Verification items for the finished model (mm, model axes). Round coordinates to 2 decimals unless told otherwise and drop trailing zeros. Order: outer loops, then holes, each group sorted by start corner. A loop starts at its lowest first (then second) coordinate and runs counter-clockwise, first axis right, second up. Notation, with made-up numbers: M 62.5,80 L 70.5,80 A27 ccw 70.5,116 Z; hole C 29.25,20 d6. An arc over 180 degrees is marked long. Write item = value, one per line. Start each with the question number.
from build123d import *


with BuildPart() as f2:
    # F2: sweep along a path in F0
    with BuildLine(Plane.XZ) as f2_path:
        Line((263.9778585136, 299.2721299103), (263.9778585136, -615.1278700897))
        Line((263.9778585136, -615.1278700897), (-345.6221414864, -615.1278700897))
        Line((-345.6221414864, -615.1278700897), (-345.6221414864, 299.2721299103))
        Line((-345.6221414864, 299.2721299103), (263.9778585136, 299.2721299103))
    # F1 (on Top) → F2 (sweep)
    with BuildSketch(Plane.XY):
        with BuildLine():
            Line((288.2001969657, -12.7), (288.2001969657, 12.7))
            Line((288.2001969657, 12.7), (281.8501969657, 12.7))
            ThreePointArc((281.8501969657, 12.7), (277.3600689052, 10.8401280605), (275.5001969657, 6.35))
            ThreePointArc((275.5001969657, 6.35), (273.6403250262, 1.8598719395), (269.1501969657, 0))
            ThreePointArc((269.1501969657, 0), (264.6600689052, -1.8598719395), (262.8001969657, -6.35))
            Line((262.8001969657, -6.35), (262.8001969657, -12.7))
            Line((262.8001969657, -12.7), (288.2001969657, -12.7))
        make_face()
    sweep(path=f2_path.line, transition=Transition.RIGHT)


solid = f2.part
1) Cross-section at B-B, the plane x = 98. Enter the section's corners in (y, z), then the cut area to 3 significant figures.
2) Cross-section at A-A, the plane z = -378.5. Enter the section's corners in (x, y), then the cut area to 3 significant figures.
3) Scan lines: probe 1 along Z at (x, y) = (210, -7.5); probe 2 along X at (y, z) = (-8, -263.5); probe 3 along Z at (x, y) = (-65, -5.25). Record each from-to range of solid material in increasing order.
Geometry results:
q1.outline = M -12.7,-639.35 L 12.7,-639.35 L 12.7,-633 A6.35 ccw 6.35,-626.65 A6.35 cw 0,-620.3 A6.35 ccw -6.35,-613.95 L -12.7,-613.95 Z; M -12.7,298.09 L -6.35,298.09 A6.35 ccw 0,304.44 A6.35 cw 6.35,310.79 A6.35 ccw 12.7,317.14 L 12.7,323.49 L -12.7,323.49 Z
q1.area = 950 mm^2
q2.outline = M -369.84,-12.7 L -344.44,-12.7 L -344.44,-6.35 A6.35 ccw -350.79,0 A6.35 cw -357.14,6.35 A6.35 ccw -363.49,12.7 L -369.84,12.7 Z; M 262.8,-12.7 L 288.2,-12.7 L 288.2,12.7 L 281.85,12.7 A6.35 ccw 275.5,6.35 A6.35 cw 269.15,0 A6.35 ccw 262.8,-6.35 Z
q2.area = 950 mm^2
q3.probe_1 = -639.35 to -613.95, 298.09 to 323.49
q3.probe_2 = -369.84 to -344.44, 262.8 to 288.2
q3.probe_3 = -639.35 to -614.05, 298.19 to 323.49
